Part model, mm, in its own coordinate system. A direction names the side the tool comes from. Round coordinates to 2 decimals unless told otherwise and drop trailing zeros. Order: outer loops, then holes, each group sorted by start corner. A loop starts at its lowest first (then second) coordinate and runs counter-clockwise, first axis right, second up. Notation, with made-up numbers: M 70.5,-8 L 103.5,-8 A29 cw 103.5,23 Z; hole C -5,72 d1. An arc over 180 degrees is marked long. One line per question, with ' | ' between items.
from build123d import *

# Parameters (mm, degrees)
F3_D     = 10
F3_DEPTH = 5
F3_TIP   = 3.0043030951
F4_DEPTH = 30


with BuildPart() as f1:
    # F0 (on Front) → F1 (revolve)
    with BuildSketch(Plane.XZ):
        with BuildLine():
            ThreePointArc((11.25, 0), (15, 3.75), (18.75, 0))
            Line((18.75, 0), (30, 0))
            Line((30, 0), (30, 7.5))
            Line((30, 7.5), (0, 7.5))
            Line((0, 7.5), (0, 0))
            Line((0, 0), (11.25, 0))
        make_face()
        with BuildLine():
            ThreePointArc((11.25, 0), (15, -3.75), (18.75, 0))
            Line((18.75, 0), (11.25, 0))
        make_face()
        with BuildLine():
            Line((11.25, 0), (18.75, 0))
            ThreePointArc((18.75, 0), (15, 3.75), (11.25, 0))
        make_face()
    revolve(axis=Axis((15, 0, 0), (1, 0, 0)))

    # F3
    with Locations(Plane(origin=(0, 0, 0), x_dir=(0, -1, 0), z_dir=(-1, 0, 0))):
        with Locations((0, 0)):
            Hole(F3_D / 2, depth=F3_DEPTH)
            with Locations((0, 0, -(F3_DEPTH + F3_TIP / 2))):  # 118° drill point
                Cone(0, F3_D / 2, F3_TIP, mode=Mode.SUBTRACT)

    # F0 (on Front) → F4 (join, symmetric)
    with BuildSketch(Plane.XZ):
        with BuildLine():
            Line((11.25, 0), (18.75, 0))
            ThreePointArc((18.75, 0), (15, 3.75), (11.25, 0))
        make_face()
        with BuildLine():
            ThreePointArc((11.25, 0), (15, -3.75), (18.75, 0))
            Line((18.75, 0), (11.25, 0))
        make_face()
    extrude(amount=F4_DEPTH, both=True)


solid = f1.part
1) Drop flat-ended pins along their axis: pin 1 (9 mm diameter, centred on y = 0, z = 0, fed in from -X); pin 2 (1.5 mm diameter, centred on y = -21, z = 3.5, fed in from +X); pin 3 (5 mm diameter, centred on y = -14.5, z = 4, fed in from +X). Give the stop position or say it passes through.
The answers:
pin 1: stops at x = 5.3 | pin 2: stops at x = 17.55 | pin 3: stops at x = 18.44
2) Saw through at B-B (x = 3). List the corners of the cut face in (y, z).
The answers:
outline: C 0,0 d15; hole C 0,0 d10
3) Saw through at D-D (z = -6.25). List the corners of the cut face in (x, y), plus the area to 3 significant figures.
The answers:
outline: M 0,-4.15 L 30,-4.15 L 30,4.15 L 0,4.15 Z | area: 249 mm²
4) Probe line 1 (Z direction, x = 2, y = 0); line 2 (X direction, y = 14.5, z = -0.25). List the from-to ranges inside material, lowest first. Write a range as [from, to].
The answers:
line 1: z = [-7.5, -5], [5, 7.5] | line 2: x = [11.26, 18.74]
5) Saw through at C-C (y = -18.5). List the corners of the cut face in (x, z).
The answers:
outline: C 15,0 d7.5
6) Two-plate mould, pull along Y, no slides. Class faces 4 (the face through (15, 30, 0)), 5 (the face through (0, 5, 2)), 6 (the face through (7.48, 0.69, -0.53)), 7 (the face through (14.79, 2.87, 6.93)): released by +Y, released by -Y, zero draft, split by the parting line, or undercut.
The answers:
face 4: released by +Y | face 5: zero draft | face 6: undercut | face 7: split by the parting line
7) Which spindle directions (+Z, -Z, +X, -X, +Y, -Y) get a long thin tool onto all of the face, cutting with end or side? Do faces 1 (the face through (18.746, 18.083, -0.165)), 2 (the face through (2.54, -1.08, -4.88)), 3 (the face through (18.746, -18.412, -0.165)). Say none if no direction does.
The answers:
face 1: +Y | face 2: -X | face 3: -Y
8) Saw through at A-A (x = 15). List the corners of the cut face in (y, z).
The answers:
outline: M -30,-3.75 L -6.5,-3.75 A7.5 ccw 6.5,-3.75 L 30,-3.75 L 30,3.75 L 6.5,3.75 A7.5 ccw -6.5,3.75 L -30,3.75 Z
